Source: CAD feature listing. Evaluate the final solid. Frame: model axes, mm. Face numbers are marked on the shaded views. A direction names the side the tool comes from. Round coordinates to 2 decimals unless told otherwise and drop trailing zeros. Order: outer loops, then holes, each group sorted by start corner. A loop starts at its lowest first (then second) coordinate and runs counter-clockwise, first axis right, second up. Notation, with made-up numbers: (61.25, 34) -> (86.25, 34) arc R24 cw to (86.25, 72) -> close; hole circle Ø2 at (77, 76.25). An arc over 180 degrees is marked (long way). One line per item, written item: value. Start each with the question number.
1) Ray query, L1, parallel to Y at x = -2.5, z = -0.8; L2, parallel to X at y = 7.25, z = 0 (3 decimals); L3, parallel to X at y = 13.5, z = 0. Return the intervals inside material, ascending.
2) Mould query, pull axis Y, two halves, no side actions, for the marked faces 1, 2, 3 and 4. Classes: pulls with the +Y half, pulls with the -Y half, needs draft (parallel to the pull), parting line crosses it, or undercut.
3) Section B-B (x = 0). Return the cut outline in (y, z) (3 decimals), and give its area (3 significant figures).
4) Section C-C (y = 12.25). Return the cut outline in (x, z), and give its area (3 significant figures).
5) Reachability of the marked faces 5, 6 and 7 from +Z, -Z, +X, -X, +Y, -Y: full face, straight path, thin tool, end or side. Return the list, or none.
6) Section D-D (y = 5.5). Return the cut outline in (x, z) (3 decimals).
7) Section A-A (z = 0). Return the cut outline in (x, y) (3 decimals).
8) Pin query (flat end, axial travel): P1, Ø1.5, axis at y = 3.5, z = -2, coming from the +X side; P2, Ø1.5, axis at x = 1.5, y = 11.5, coming from the +Z side. Return the tip coordinate at first contact, or that it passes through.
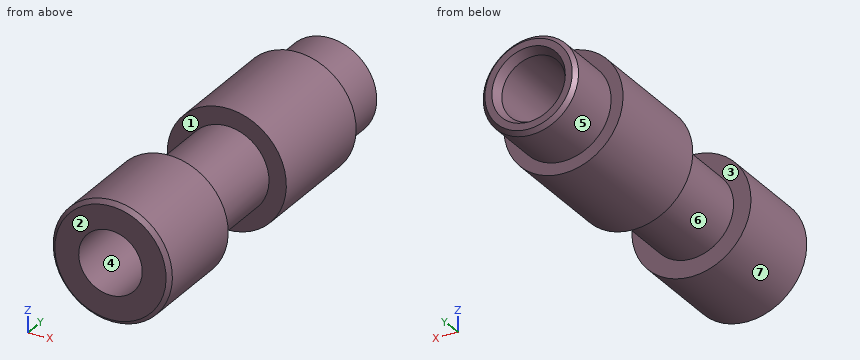
```python
from build123d import *

# Parameters (mm, degrees)
CHAFL_N4_SIZE  = 0.2
CHAFL_N5_SIZE  = 0.25
CHAFL_N5_SIZE2 = 0.433012702


with BuildPart() as part:
    # Croquis3 → Revolución1 (revolve)
    with BuildSketch(Plane.XY, mode=Mode.PRIVATE) as revoluci_n1_sk:
        Polygon((-1.6, 0), (-1.6, 19), (-2.4, 19), (-2.4, 16), (-3, 16), (-3, 10), (-2.125, 10), (-2.125, 5), (-3, 5), (-3, 0), align=None)
    revolve(revoluci_n1_sk.sketch.rotate(Axis((0, 0, 0), (0, 1, 0)), 270), axis=Axis((0, 0, 0), (0, 1, 0)))

    # Chaflán4
    chafl_n4_edges = [part.edges().sort_by_distance(p)[0] for p in [
        (0, 19, 2.4),
        (0, 0, 3),
    ]]
    chamfer(chafl_n4_edges, length=CHAFL_N4_SIZE)

    # Chaflán5
    chafl_n5_edges = [part.edges().sort_by_distance(p)[0] for p in [
        (0, 19, 1.6),
    ]]
    chafl_n5_side = [part.faces().sort_by_distance(p)[0] for p in [
        (0, 19, 2.137774603),
    ]]
    chamfer(chafl_n5_edges, length=CHAFL_N5_SIZE, length2=CHAFL_N5_SIZE2, reference=chafl_n5_side[0])


solid = part.part
```
Findings:
1. L1: 0 to 5, 10 to 16
1. L2: -2.125 to -1.6, 1.6 to 2.125
1. L3: -3 to -1.6, 1.6 to 3
2. face 1: undercut
2. face 2: pulls with the -Y half
2. face 3: undercut
2. face 4: needs draft
3. outline: (0, -2.8) -> (0.2, -3) -> (5, -3) -> (5, -2.125) -> (10, -2.125) -> (10, -3) -> (16, -3) -> (16, -2.4) -> (18.8, -2.4) -> (19, -2.2) -> (19, -1.85) -> (18.567, -1.6) -> (0, -1.6) -> close; (0, 1.6) -> (18.567, 1.6) -> (19, 1.85) -> (19, 2.2) -> (18.8, 2.4) -> (16, 2.4) -> (16, 3) -> (10, 3) -> (10, 2.125) -> (5, 2.125) -> (5, 3) -> (0.2, 3) -> (0, 2.8) -> close
3. area: 40.7 mm2
4. outline: circle Ø6 at (0, 0); hole circle Ø3.2 at (0, 0)
4. area: 20.2 mm2
5. face 5: +Y
5. face 6: none
5. face 7: +Y, -Y
6. outline: circle Ø4.25 at (0, 0); hole circle Ø3.2 at (0, 0)
7. outline: (-3, 0.2) -> (-2.8, 0) -> (-1.6, 0) -> (-1.6, 18.567) -> (-1.85, 19) -> (-2.2, 19) -> (-2.4, 18.8) -> (-2.4, 16) -> (-3, 16) -> (-3, 10) -> (-2.125, 10) -> (-2.125, 5) -> (-3, 5) -> close; (1.6, 0) -> (2.8, 0) -> (3, 0.2) -> (3, 5) -> (2.125, 5) -> (2.125, 10) -> (3, 10) -> (3, 16) -> (2.4, 16) -> (2.4, 18.8) -> (2.2, 19) -> (1.85, 19) -> (1.6, 18.567) -> close
8. P1: x = 2.73
8. P2: z = 2.9
